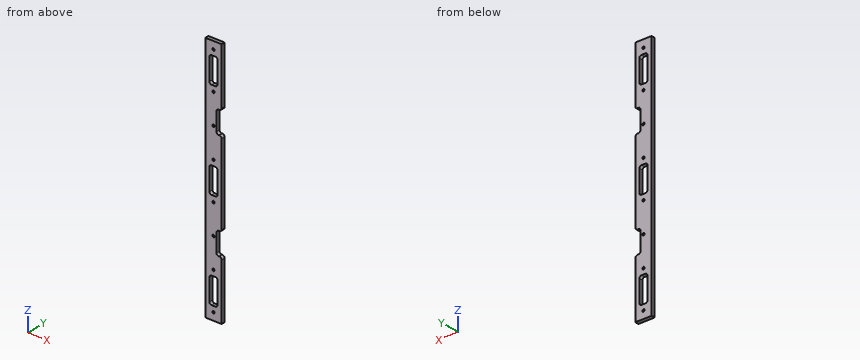
```python
from build123d import *

# Parameters (mm, degrees)
SKETCH_1_W          = 22
SKETCH_1_H          = 330
SKETCH_1_R          = 1.55
EXTRUDE_1_DEPTH     = 5
SKETCH_2_W          = 14
SKETCH_2_H          = 30
CUT_EXTRUDE_1_DEPTH = 166.441832678
FILLET_1_R          = 3
SKETCH_3_W          = 11
SKETCH_3_H          = 35
CUT_EXTRUDE_2_DEPTH = 166.441832678
FILLET_2_R          = 3


with BuildPart() as part:
    # 草图1 → 凸台-拉伸1 (new body)
    with BuildSketch(Plane(origin=(0, 0, 0), x_dir=(1, 0, 0), z_dir=(0, 1, 0))):
        Rectangle(SKETCH_1_W, SKETCH_1_H)
        with Locations(Location((0, 25, 0), (0, 0, 270))):
            Circle(SKETCH_1_R, mode=Mode.SUBTRACT)
        with Locations(Location((0, 65, 0), (0, 0, 270))):
            Circle(SKETCH_1_R, mode=Mode.SUBTRACT)
        with Locations(Location((0, -25, 0), (0, 0, 90))):
            Circle(SKETCH_1_R, mode=Mode.SUBTRACT)
        with Locations(Location((0, -65, 0), (0, 0, 90))):
            Circle(SKETCH_1_R, mode=Mode.SUBTRACT)
        with Locations(Location((0, 105, 0), (0, 0, 270))):
            Circle(SKETCH_1_R, mode=Mode.SUBTRACT)
        with Locations(Location((0, 155, 0), (0, 0, 270))):
            Circle(SKETCH_1_R, mode=Mode.SUBTRACT)
        with Locations(Location((0, -155, 0), (0, 0, 90))):
            Circle(SKETCH_1_R, mode=Mode.SUBTRACT)
        with Locations(Location((0, -105, 0), (0, 0, 90))):
            Circle(SKETCH_1_R, mode=Mode.SUBTRACT)
    extrude(amount=EXTRUDE_1_DEPTH)

    # 草图2 → 切除-拉伸1 (cut, through all)
    with BuildSketch(Plane(origin=(0, 5, 0), x_dir=(1, 0, 0), z_dir=(0, 1, 0))):
        with Locations((11, 71.5)):
            Rectangle(SKETCH_2_W, SKETCH_2_H)
        with Locations((11, -71.5)):
            Rectangle(SKETCH_2_W, SKETCH_2_H)
    extrude(amount=-CUT_EXTRUDE_1_DEPTH, mode=Mode.SUBTRACT)

    # 圆角1
    fillet_1_edges = [part.edges().sort_by_distance(p)[0] for p in [
        (11, 2.5, 86.5),
        (11, 2.5, 56.5),
        (11, 2.5, -86.5),
        (11, 2.5, -56.5),
        (4, 2.5, -86.5),
        (4, 2.5, -56.5),
        (4, 2.5, 56.5),
        (4, 2.5, 86.5),
    ]]
    fillet(fillet_1_edges, radius=FILLET_1_R)

    # 草图3 → 切除-拉伸2 (cut, through all)
    with BuildSketch(Plane(origin=(0, 5, 0), x_dir=(1, 0, 0), z_dir=(0, 1, 0))):
        with Locations((0, 130)):
            Rectangle(SKETCH_3_W, SKETCH_3_H)
        with Locations((0, -130)):
            Rectangle(SKETCH_3_W, SKETCH_3_H)
        Rectangle(SKETCH_3_W, SKETCH_3_H)
    extrude(amount=-CUT_EXTRUDE_2_DEPTH, mode=Mode.SUBTRACT)

    # 圆角2
    fillet_2_edges = [part.edges().sort_by_distance(p)[0] for p in [
        (5.5, 2.5, -147.5),
        (5.5, 2.5, -112.5),
        (-5.5, 2.5, -112.5),
        (-5.5, 2.5, -147.5),
        (-5.5, 2.5, 147.5),
        (-5.5, 2.5, 112.5),
        (5.5, 2.5, 112.5),
        (5.5, 2.5, 147.5),
        (5.5, 2.5, -17.5),
        (5.5, 2.5, 17.5),
        (-5.5, 2.5, 17.5),
        (-5.5, 2.5, -17.5),
    ]]
    fillet(fillet_2_edges, radius=FILLET_2_R)


solid = part.part
```
Geometry: final body of the model. Coordinates: model frame, mm. Coordinates: 2 decimals unless noted, no trailing zeros. Write each loop counter-clockwise with the first axis right and the second up, starting at its lowest first coordinate (ties: lowest second). Pieces come first, ordered by that corner, then holes. Notation, with made-up numbers: M -32,-33.75 L -4,-33.75 A22 ccw -4,-5.75 Z; hole C 25,27 d4. An arc over 180 degrees is marked long. Answer as CSV lines item,"result". Start each with the question number.
Q1. Line query: line 1 (Z direction, x = 6.75, y = 4.75); line 2 (Z direction, x = -5, y = 4.35); line 3 (X direction, y = 1.3, z = -65). Output: solid intervals per line, ascending. Write a range as from..to.
Q2. Cut plane B-B on y = 3.8. Count the separate pieces of the cut face and the enclosed holes in it, then the cut area to 3 significant figures.
Q3. Pin query (flat end, axial travel): P1, Ø3, axis at x = 0, z = -25, coming from the -Y side; P2, Ø1.5, axis at y = 1.5, z = -70.5, coming from the +X side. Return the tip coordinate at first contact, or that it passes through.
Q4. Cut plane A-A on z = 11. Return the cut outline in (x, y), then the cut area to 3 significant figures.
Findings below:
1,line 1,"z = -165..-86.49, -56.51..56.51, 86.49..165"
1,line 2,"z = -165..-146.16, -113.84..-16.16, 16.16..113.84, 146.16..165"
1,line 3,"x = -11..-1.55, 1.55..4"
2,separate pieces,"1"
2,enclosed holes,"11"
2,area,"5,650 mm2"
3,P1,"passes through"
3,P2,"stops at x = 4"
4,outline,"M -11,0 L -5.5,0 L -5.5,5 L -11,5 Z; M 5.5,0 L 11,0 L 11,5 L 5.5,5 Z"
4,area,"55.0 mm2"
